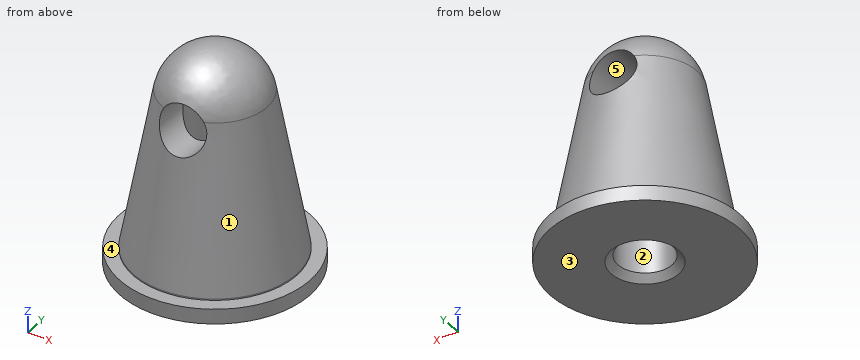
Autodesk Inventor part; units mm, degrees
ref_plane "Work Plane1" through (0, 0, 16.1) normal (0, 0, 1) x (1, 0, 0)
ref_plane "YZ Plane" through (0, 0, 0) normal (1, 0, 0) x (0, 1, 0)
ref_plane "XZ Plane" through (0, 0, 0) normal (0, 1, 0) x (-1, 0, 0)
sketch "Sketch1" plane through (0, 0, 0) normal (0, 0, 1) x (1, 0, 0)
  circle A0 centre (0, 0) radius 7
  dimension "d0" = 14
extrude "Extrusion1" add sketch "Sketch1" along normal blind 1.1
sketch "Sketch2" plane through (0, 0, 1.1) normal (0, 0, 1) x (1, 0, 0)
  circle A0 centre (0, 0) radius 7
  circle A1 centre (0, 0) radius 6
  dimension "d3" = 12
ref_plane "Work Plane1" through (0, 0, 16.1) normal (0, 0, 1) x (1, 0, 0)
sketch "Sketch3" plane through (0, 0, 16.1) normal (0, 0, 1) x (1, 0, 0)
  circle A0 centre (0, 0) radius 3.25
  dimension "d5" = 6.5
extrude "Extrusion2" add sketch "Sketch2" along normal blind 0.1 contours A1
loft "Loft1" add profiles "Sketch3" section 1 edges at (-6, 0, 1.2)
fillet "Fillet1" radius 3.9 1 edges at (-3.25, 0, 16.1)
sketch "Sketch4" plane through (0, 0, 0) normal (0, 1, 0) x (-1, 0, 0)
  circle A0 centre (0, 12) radius 1.75
  point P0 (0, 0)
  dimension "d13" = 12
  dimension "d14" = 3.5
extrude "Extrusion3" cut sketch "Sketch4" along normal through all both and the other way through all
sketch "Sketch5" plane through (0, 0, 0) normal (0, 0, -1) x (-1, 0, 0)
  circle A0 centre (0, 0) radius 7
  circle A1 centre (0, 0) radius 2
  dimension "d17" = 4
extrude "Extrusion4" cut sketch "Sketch5" against normal blind 12 contours A1
chamfer "Chamfer1" distance 0.5 angle 45 1 edges at (2, 0, 0)
properties part number "nut"
For this review, take the finished solid that the model builds, in its own axes (mm). Face numbers are marked on the shaded views. A direction names the side the tool comes from. Give positions to 0.01 mm unless a question says otherwise; leave off trailing zeros. Order: outer loops, then holes, each group sorted by start corner. A loop starts at its lowest first (then second) coordinate and runs counter-clockwise, first axis right, second up.
1) For the marked faces 4 and 5, list the 3-axis set-ups (+Z, -Z, +X, -X, +Y, -Y) from which the entire face can be reached by the end or side of a thin tool; tool diameter is ignored.
2) The part is to be moulded in two halves that separate along X. For the marked faces 1, 2 and 3, say which applies: released by +X, released by -X, zero draft, split by the parting line, or undercut.
3) Take a section at A-A (x = 1.25). State how many separate pieces and enclosed holes the cut face has, then the cut area to 3 significant figures.
4) Take a section at C-C (z = 7.25). Give the boundary of the cut face in (x, y), then the cut area to 3 significant figures.
5) Insertion check: pin 1 (3 mm diameter, centred on x = 2.5, y = 3.5, fed in from +Z); pin 2 (6 mm diameter, centred on y = -5.5, z = 8, fed in from +X); pin 3 (4 mm diameter, centred on x = -2.5, y = 3.5, fed in from +Z); pin 4 (1.5 mm diameter, centred on x = 0.5, y = -4.5, fed in from -Z). Each pin has a flat end and moves straight along its axis. Give the tip position at first contact, or say it passes through.
6) Take a section at B-B (z = 10). Give the boundary of the cut face in (x, y).
7) Wall thickness on line 1 (X direction, y = 1.25, z = 12); line 2 (Z direction, x = 4, y = 5.5); line 3 (Y direction, x = -1, z = 10): over which ranges is each line inside the solid? List them lowest first.
Derived:
1. face 4: +Z
1. face 5: +Y, -Y
2. face 1: split by the parting line
2. face 2: undercut
2. face 3: zero draft
3. separate pieces: 3
3. enclosed holes: 0
3. area: 91.3 mm2
4. outline: circle Ø9.77 at (0, 0); hole circle Ø4 at (0, 0)
4. area: 62.4 mm2
5. pin 1: stops at z = 14.92
5. pin 2: stops at x = 4.14
5. pin 3: stops at z = 15.35
5. pin 4: stops at z = 0
6. outline: circle Ø8.75 at (0, 0); hole circle Ø4 at (0, 0)
7. line 1: x = -3.81 to -1.75, 1.75 to 3.81
7. line 2: z = 0 to 1.1
7. line 3: y = -4.26 to -1.73, 1.73 to 4.26
